Could you check a few things on this model? Use its own coordinates, in mm. Face numbers are marked on the shaded views. A direction names the side the tool comes from. Coordinates: 2 decimals unless noted, no trailing zeros. Order: outer loops, then holes, each group sorted by start corner. A loop starts at its lowest first (then second) coordinate and runs counter-clockwise, first axis right, second up. Notation, with made-up numbers: M 73,32 L 109,32 A25 ccw 109,67 Z; hole C -0.5,27 d2. An arc over 180 degrees is marked long. Write item = value, one per line. Start each with the question number.
from build123d import *

# Parameters (mm, degrees)
BOSS_EXTRUDE1_DEPTH      = 6
BOSS_EXTRUDE2_DEPTH      = 40
CUT_EXTRUDE1_REACH       = 62.762
SKETCH9_R                = 1.5
CUT_EXTRUDE2_REACH       = 62.762
SKETCH10_R               = 7
BOSS_EXTRUDE4_DEPTH      = 25
BOSS_EXTRUDE5_REACH      = 73.576
BOSS_EXTRUDE5_END_RADIUS = 23.4
SKETCH12_R               = 2.5
BOSS_EXTRUDE6_REACH      = 73.576
SKETCH14_R               = 2.5
SKETCH15_W               = 42.894850158
SKETCH15_H               = 27.148059605
CUT_EXTRUDE3_DEPTH       = 6
FILLET1_R                = 2
SKETCH7_R                = 4
CUT_EXTRUDE4_DEPTH       = 3


with BuildPart() as part:
    # Sketch3 → Boss-Extrude1 (new body)
    with BuildSketch(Plane.XY):
        with BuildLine():
            Line((-20, 10.240601504), (20, 10.240601504))
            ThreePointArc((20, 10.240601504), (24.242640687, 8.483242191), (26, 4.240601504))
            Line((26, 4.240601504), (26, -13.759398496))
            ThreePointArc((26, -13.759398496), (24.242640687, -18.002039183), (20, -19.759398496))
            Line((20, -19.759398496), (-20, -19.759398496))
            ThreePointArc((-20, -19.759398496), (-24.242640687, -18.002039183), (-26, -13.759398496))
            Line((-26, -13.759398496), (-26, 4.240601504))
            ThreePointArc((-26, 4.240601504), (-24.242640687, 8.483242191), (-20, 10.240601504))
        make_face()
    extrude(amount=BOSS_EXTRUDE1_DEPTH)

    # Sketch4 → Boss-Extrude2 (add)
    with BuildSketch(Plane.XY.offset(6)):
        with BuildLine():
            Line((-26, 4.240601504), (26, 4.240601504))
            ThreePointArc((26, 4.240601504), (24.242640687, 8.483242191), (20, 10.240601504))
            Line((20, 10.240601504), (-20, 10.240601504))
            ThreePointArc((-20, 10.240601504), (-24.242640687, 8.483242191), (-26, 4.240601504))
        make_face()
    extrude(amount=BOSS_EXTRUDE2_DEPTH)

    # Sketch9 → Cut-Extrude1 (cut, up to next)
    with BuildSketch(Plane(origin=(0, 10.240601504, 0), x_dir=(1, 0, 0), z_dir=(0, 1, 0)), mode=Mode.PRIVATE) as cut_extrude1_sk1:
        with Locations(Location((0, -41.5, 0), (0, 0, 180))):
            Circle(SKETCH9_R)
    cut_extrude1_tool1 = extrude(cut_extrude1_sk1.sketch, amount=-CUT_EXTRUDE1_REACH, mode=Mode.PRIVATE) & part.part
    # Sketch9 → Cut-Extrude1 (cut, up to next)
    with BuildSketch(Plane(origin=(0, 10.240601504, 0), x_dir=(1, 0, 0), z_dir=(0, 1, 0)), mode=Mode.PRIVATE) as cut_extrude1_sk2:
        with Locations(Location((13.423393759, -33.75, 0), (0, 0, 180))):
            Circle(SKETCH9_R)
    cut_extrude1_tool2 = extrude(cut_extrude1_sk2.sketch, amount=-CUT_EXTRUDE1_REACH, mode=Mode.PRIVATE) & part.part
    # Sketch9 → Cut-Extrude1 (cut, up to next)
    with BuildSketch(Plane(origin=(0, 10.240601504, 0), x_dir=(1, 0, 0), z_dir=(0, 1, 0)), mode=Mode.PRIVATE) as cut_extrude1_sk3:
        with Locations(Location((-13.423393759, -33.75, 0), (0, 0, 180))):
            Circle(SKETCH9_R)
    cut_extrude1_tool3 = extrude(cut_extrude1_sk3.sketch, amount=-CUT_EXTRUDE1_REACH, mode=Mode.PRIVATE) & part.part
    # Sketch9 → Cut-Extrude1 (cut, up to next)
    with BuildSketch(Plane(origin=(0, 10.240601504, 0), x_dir=(1, 0, 0), z_dir=(0, 1, 0)), mode=Mode.PRIVATE) as cut_extrude1_sk4:
        with Locations(Location((-13.423393759, -18.25, 0), (0, 0, 180))):
            Circle(SKETCH9_R)
    cut_extrude1_tool4 = extrude(cut_extrude1_sk4.sketch, amount=-CUT_EXTRUDE1_REACH, mode=Mode.PRIVATE) & part.part
    # Sketch9 → Cut-Extrude1 (cut, up to next)
    with BuildSketch(Plane(origin=(0, 10.240601504, 0), x_dir=(1, 0, 0), z_dir=(0, 1, 0)), mode=Mode.PRIVATE) as cut_extrude1_sk5:
        with Locations(Location((0, -10.5, 0), (0, 0, 180))):
            Circle(SKETCH9_R)
    cut_extrude1_tool5 = extrude(cut_extrude1_sk5.sketch, amount=-CUT_EXTRUDE1_REACH, mode=Mode.PRIVATE) & part.part
    # Sketch9 → Cut-Extrude1 (cut, up to next)
    with BuildSketch(Plane(origin=(0, 10.240601504, 0), x_dir=(1, 0, 0), z_dir=(0, 1, 0)), mode=Mode.PRIVATE) as cut_extrude1_sk6:
        with Locations(Location((13.423393759, -18.25, 0), (0, 0, 180))):
            Circle(SKETCH9_R)
    cut_extrude1_tool6 = extrude(cut_extrude1_sk6.sketch, amount=-CUT_EXTRUDE1_REACH, mode=Mode.PRIVATE) & part.part
    add(cut_extrude1_tool1.solids().sort_by_distance((0, 10.240602, 41.5))[0], mode=Mode.SUBTRACT)
    add(cut_extrude1_tool2.solids().sort_by_distance((13.423394, 10.240602, 33.75))[0], mode=Mode.SUBTRACT)
    add(cut_extrude1_tool3.solids().sort_by_distance((-13.423394, 10.240602, 33.75))[0], mode=Mode.SUBTRACT)
    add(cut_extrude1_tool4.solids().sort_by_distance((-13.423394, 10.240602, 18.25))[0], mode=Mode.SUBTRACT)
    add(cut_extrude1_tool5.solids().sort_by_distance((0, 10.240602, 10.5))[0], mode=Mode.SUBTRACT)
    add(cut_extrude1_tool6.solids().sort_by_distance((13.423394, 10.240602, 18.25))[0], mode=Mode.SUBTRACT)

    # Sketch10 → Cut-Extrude2 (cut, up to next)
    with BuildSketch(Plane(origin=(0, 10.240601504, 0), x_dir=(1, 0, 0), z_dir=(0, 1, 0)), mode=Mode.PRIVATE) as cut_extrude2_sk1:
        with Locations(Location((7.059090501, -26, 0), (0, 0, 180))):
            Circle(SKETCH10_R)
    cut_extrude2_tool1 = extrude(cut_extrude2_sk1.sketch, amount=-CUT_EXTRUDE2_REACH, mode=Mode.PRIVATE) & part.part
    add(cut_extrude2_tool1.solids().sort_by_distance((7.059091, 10.240602, 26))[0], mode=Mode.SUBTRACT)

    # Sketch11 → Boss-Extrude4 (add)
    with BuildSketch(Plane(origin=(0, 10.240601504, 0), x_dir=(1, 0, 0), z_dir=(0, 1, 0))):
        with BuildLine():
            Line((16.710143733, -16.95726278), (20.169460133, -14.136068192))
            ThreePointArc((20.169460133, -14.136068192), (0.449710611, -2.604321759), (-19.698633669, -13.369725595))
            Line((-19.698633669, -13.369725595), (-16.193668166, -16.061936238))
            ThreePointArc((-16.193668166, -16.061936238), (0.516806692, -7.007029963), (16.710143733, -16.95726278))
        make_face()
    extrude(amount=BOSS_EXTRUDE4_DEPTH)

    # Boss-Extrude5: up to this cylinder (the profile starts outside it)
    boss_extrude5_end = Plane(origin=(0, 6.683051, 26), z_dir=(0, -1, 0)) * Cylinder(BOSS_EXTRUDE5_END_RADIUS, 194.952, mode=Mode.PRIVATE)
    # Sketch12 → Boss-Extrude5 (add, up to the surface)
    with BuildSketch(Plane(origin=(7.879699248, -7.879699248, 0), x_dir=(0, 0, 1), z_dir=(-0.7071067811865489, 0.7071067811865462, 0)), mode=Mode.PRIVATE) as boss_extrude5_sk1:
        with Locations((7.574761701, 20.594839086)):
            Circle(SKETCH12_R)
    boss_extrude5_tool1 = extrude(boss_extrude5_sk1.sketch, amount=BOSS_EXTRUDE5_REACH, mode=Mode.PRIVATE) - boss_extrude5_end
    add(boss_extrude5_tool1.solids().sort_by_distance((22.44245, 6.683051, 7.574762))[0])

    # Sketch14 → Boss-Extrude6 (add, up to next)
    with BuildSketch(Plane(origin=(-7.879699248, -7.879699248, 0), x_dir=(0, 0, -1), z_dir=(0.7071067811865487, 0.7071067811865465, 0)), mode=Mode.PRIVATE) as boss_extrude6_sk1:
        with Locations((-10.283332747, 20.780524406)):
            Circle(SKETCH14_R)
    boss_extrude6_tool1 = extrude(boss_extrude6_sk1.sketch, amount=BOSS_EXTRUDE6_REACH, mode=Mode.PRIVATE) - part.part
    add(boss_extrude6_tool1.solids().sort_by_distance((-22.573749, 6.81435, 10.283333))[0])

    # Sketch15 → Cut-Extrude3 (cut)
    with BuildSketch(Plane(origin=(0, 0, 0), x_dir=(-1, 0, 0), z_dir=(0, 0, -1))):
        with Locations((-27.245771634, -9.333428299)):
            Rectangle(SKETCH15_W, SKETCH15_H)
    extrude(amount=-CUT_EXTRUDE3_DEPTH, mode=Mode.SUBTRACT)

    # Fillet1
    fillet1_edges = [part.edges().sort_by_distance(p)[0] for p in [
        (5.798346555, -19.759398496, 3),
        (5.798346555, 4.240601504, 3),
    ]]
    fillet(fillet1_edges, radius=FILLET1_R)

    # Sketch7 → Cut-Extrude4 (cut)
    with BuildSketch(Plane(origin=(0, 0, 0), x_dir=(-1, 0, 0), z_dir=(0, 0, -1))):
        with Locations((0, -4.759398496)):
            Circle(SKETCH7_R)
    extrude(amount=-CUT_EXTRUDE4_DEPTH, mode=Mode.SUBTRACT)


solid = part.part
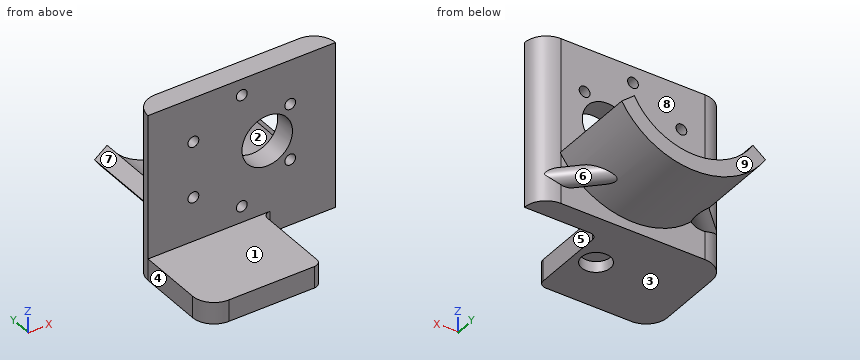
(1) Imagine slicing it at B-B on z = 41.5. List the corners of the cut face in (x, y) for me.
(2) For the marked faces 1, 2, 3, 4 and 5, which set-ups out of +Z, -Z, +X, -X, +Y, -Y let a thin tool reach every point of the face, with its end or its side?
(3) Will these pins go through, and if not, where does the flat tip stop? P1, Ø4, axis at y = 8.5, z = 6, coming from the +X side; P2, Ø8.5, axis at x = 7.06, z = 26, coming from the +Y side; P3, Ø2, axis at x = -8, z = 21.5, coming from the -Y side; P4, Ø5, axis at y = -5.5, z = 2.5, coming from the +X side.
(4) Thinking about a two-plate mould opening in X: for the marked faces 6, 7, 8 and 9, which applies, released by +X, released by -X, zero draft, split by the parting line, or undercut?
(5) Imagine slicing it at A-A on z = 18.25. List the corners of the cut face in (x, y) for me.
(6) Please list where these lines run through material, in increasing order: probe 1 along Z at (x, y) = (0, 6.5); probe 2 along X at (y, z) = (5.5, 18); probe 3 along Z at (x, y) = (13.5, 6). Write a range as from..to.
(7) Imagine slicing it at C-C on y = 6. List the corners of the cut face in (x, z) for me, plus the area to 3 significant figures.
(8) Imagine slicing it at D-D on x = -8.5. List the corners of the cut face in (y, z) for me.
Response:
q1.outline = M -26,4.24 L -1.5,4.24 L -1.5,10.24 L -20,10.24 A6 ccw Z; M 1.5,4.24 L 26,4.24 A6 ccw 20,10.24 L 1.5,10.24 Z
q2.face_1 = +Z, +X, -X, -Y
q2.face_2 = +Z, +Y
q2.face_3 = -Z, +X, -X, +Y, -Y
q2.face_4 = +Z, -Z, -X, +Y, -Y
q2.face_5 = +Z, -Z, +X, -Y
q3.P1 = 25.56
q3.P2 = through
q3.P3 = 4.24
q3.P4 = 5.8
q4.face_6 = undercut
q4.face_7 = released by -X
q4.face_8 = undercut
q4.face_9 = zero draft
q5.outline = M -26,4.24 L -14.92,4.24 L -14.92,10.24 L -20,10.24 A6 ccw Z; M -11.92,4.24 L 11.92,4.24 L 11.92,10.24 L -11.92,10.24 Z; M 14.92,4.24 L 26,4.24 A6 ccw 20,10.24 L 14.92,10.24 Z
q6.probe_1 = 0..9, 12..40, 43..46
q6.probe_2 = -25.87..-14.9, -11.94..11.94, 14.9..25.87
q6.probe_3 = 0..16.75, 19.75..23.26, 28.74..32.25, 35.25..46
q7.outline = M -25.74,0 L 25.74,0 L 25.74,46 L -25.74,46 Z; hole C -13.42,18.25 d3; hole C -13.42,33.75 d3; hole C 0,10.5 d3; hole C 0,41.5 d3; hole C 7.06,26 d14; hole C 13.42,18.25 d3; hole C 13.42,33.75 d3
q7.area = 2,170 mm2
q8.outline = M -19.76,0 L 10.24,0 L 10.24,4.2 L 35.24,4.2 L 35.24,9.01 L 10.24,9.01 L 10.24,46 L 4.24,46 L 4.24,6 L -19.76,6 Z
